Work out the finished part from the listing and answer in its coordinate system (mm). A direction names the side the tool comes from. Coordinates: 2 decimals unless noted, no trailing zeros. Loops run counter-clockwise (first coordinate to the right, second up) from the corner with the lowest first, then second, coordinate; pieces in that order, holes last. Notation, with made-up numbers: (35.25, 18.25) - (56.25, 18.25) arc R31 ccw to (56.25, 50.25) - close; hole circle Ø5 at (72, 0). An arc over 180 degrees is marked (long way). Write each question's results on one line, items separated by ' | '. Start each with the question number.
Item 1: Section A-A, the plane z = 37.5 is taken. Write down the section's boundary in (x, y).
Item 2: A tool of negligible diameter and unlimited length cuts with its end or side. For faces 4 (the face through (35, -13, 12.7)), 5 (the face through (6, -6.354, 38)), 6 (the face through (17, 0, 9)), from which of +Z, -Z, +X, -X, +Y, -Y can it reach the whole face along a straight path? Write none if from no direction.
Item 3: Consider probe 1 along X at (y, z) = (-11.75, 5); probe 2 along X at (y, z) = (-8, 8); probe 3 along Z at (x, y) = (34.5, -6.75). Determine where each line is inside the solid, lowest interval first. Write a range as [from, to].
Item 4: For a pull along Y with two mould halves and no side action, classify faces 1 (the face through (6, -19.046, 37)), 2 (the face through (6.439, -1.802, 38.489)), 3 (the face through (0, -13, 17)) as +Y half, -Y half, draft (parallel to the pull), parting line (faces both ways), or undercut.
Item 5: Section D-D, the plane x = 15.5 is taken. Write down the section's boundary in (y, z), plus the area to 3 significant figures.
Item 6: Section C-C, the plane z = 6 is taken. Write down the section's boundary in (x, y), plus the area to 3 significant figures.
Item 7: Each of these flat-tipped pins is pushed along its axis until it touches: pin 1 Ø4 at (y, z) = (-9, 18.5) entering from +X; pin 2 Ø12 at (x, z) = (6, 36.5) entering from -Y; pin 3 Ø5.5 at (x, z) = (5.5, 40) entering from +Y; pin 4 Ø8 at (y, z) = (-12.5, 37.5) entering from -X. Where does it stop, or does it pass through?
Item 8: Section B-B, the plane y = -11 is taken. Write down the section's boundary in (x, z), plus the area to 3 significant figures.
from build123d import *

# Parameters (mm, degrees)
F1_DEPTH = 25.4
F3_DEPTH = 12.701
F5_DEPTH = 12.701
F7_DEPTH = 57.151


with BuildPart() as f1:
    # F0 (on Front) → F1 (new body)
    with BuildSketch(Plane.XZ):
        Polygon((0, 44.45), (0, 0), (57.15, 0), (57.15, 12.7), (12.7, 12.7), (12.7, 44.45), align=None)
    extrude(amount=F1_DEPTH)

    # F2 (on face) → F3 (cut, through all)
    with BuildSketch(Plane.XY.offset(12.7)):
        with BuildLine():
            Line((25.4, -19.05), (25.4, -6.35))
            ThreePointArc((25.4, -6.35), (19.05, -12.7), (25.4, -19.05))
        make_face()
        with BuildLine():
            ThreePointArc((31.75, -12.7), (29.8901280605, -8.2098719395), (25.4, -6.35))
            Line((25.4, -6.35), (25.4, -19.05))
            ThreePointArc((25.4, -19.05), (29.8901280605, -17.1901280605), (31.75, -12.7))
        make_face()
        with BuildLine():
            Line((44.45, -19.05), (44.45, -6.35))
            ThreePointArc((44.45, -6.35), (38.1, -12.7), (44.45, -19.05))
        make_face()
        with BuildLine():
            ThreePointArc((50.8, -12.7), (48.9401280605, -8.2098719395), (44.45, -6.35))
            Line((44.45, -6.35), (44.45, -19.05))
            ThreePointArc((44.45, -19.05), (48.9401280605, -17.1901280605), (50.8, -12.7))
        make_face()
        with BuildLine():
            Line((57.15, 0), (44.45, 0))
            ThreePointArc((44.45, 0), (53.4302561211, -3.7197438789), (57.15, -12.7))
            Line((57.15, -12.7), (57.15, 0))
        make_face()
        with BuildLine():
            Line((57.15, -25.4), (57.15, -12.7))
            ThreePointArc((57.15, -12.7), (53.4302561211, -21.6802561211), (44.45, -25.4))
            Line((44.45, -25.4), (57.15, -25.4))
        make_face()
    extrude(amount=-F3_DEPTH, mode=Mode.SUBTRACT)

    # F4 (on face) → F5 (cut, through all)
    with BuildSketch(Plane.YZ.offset(12.7)):
        with BuildLine():
            ThreePointArc((-25.4, 32.1787146746), (-25.4018088896, 31.9643573373), (-25.4, 31.75))
            Line((-25.4, 31.75), (-25.4, 32.1787146746))
        make_face()
        with BuildLine():
            Line((0, 32.1787146746), (0, 31.75))
            ThreePointArc((0, 31.75), (0.0018088896, 31.9643573373), (0, 32.1787146746))
        make_face()
        with BuildLine():
            Line((-25.4, 44.45), (-25.4, 32.1787146746))
            ThreePointArc((-25.4, 32.1787146746), (-22.4029254465, 40.1612583888), (-15.0333830306, 44.45))
            Line((-15.0333830306, 44.45), (-25.4, 44.45))
        make_face()
        with BuildLine():
            ThreePointArc((-10.3666169694, 44.45), (-2.9970745535, 40.1612583888), (0, 32.1787146746))
            Line((0, 32.1787146746), (0, 44.45))
            Line((0, 44.45), (-10.3666169694, 44.45))
        make_face()
    extrude(amount=-F5_DEPTH, mode=Mode.SUBTRACT)

    # F6 (on face) → F7 (cut, through all)
    with BuildSketch(Plane(origin=(0, 0, 0), x_dir=(0, -1, 0), z_dir=(-1, 0, 0))):
        with BuildLine():
            Line((6.3536190682, 32.1787146746), (6.3536190682, 31.75))
            Line((6.3536190682, 31.75), (19.0463809318, 31.75))
            Line((19.0463809318, 31.75), (19.0463809318, 32.1787146746))
            ThreePointArc((19.0463809318, 32.1787146746), (12.7, 38.3143573373), (6.3536190682, 32.1787146746))
        make_face()
        with BuildLine():
            Line((19.0463809318, 31.75), (6.3536190682, 31.75))
            ThreePointArc((6.3536190682, 31.75), (12.7, 25.6143573373), (19.0463809318, 31.75))
        make_face()
        with BuildLine():
            ThreePointArc((6.3536190682, 32.1787146746), (6.35, 31.9643573373), (6.3536190682, 31.75))
            Line((6.3536190682, 31.75), (6.3536190682, 32.1787146746))
        make_face()
        with BuildLine():
            Line((19.0463809318, 32.1787146746), (19.0463809318, 31.75))
            ThreePointArc((19.0463809318, 31.75), (19.0490951685, 31.8571633942), (19.05, 31.9643573373))
            ThreePointArc((19.05, 31.9643573373), (19.0490951685, 32.0715512803), (19.0463809318, 32.1787146746))
        make_face()
        with BuildLine():
            Line((6.3536190682, 42.9670569213), (6.3536190682, 32.1787146746))
            ThreePointArc((6.3536190682, 32.1787146746), (12.7, 38.3143573373), (19.0463809318, 32.1787146746))
            Line((19.0463809318, 32.1787146746), (19.0463809318, 42.9670569213))
            ThreePointArc((19.0463809318, 42.9670569213), (17.1027668181, 43.8787013567), (15.0333830306, 44.45))
            Line((15.0333830306, 44.45), (10.3666169694, 44.45))
            ThreePointArc((10.3666169694, 44.45), (8.2972331819, 43.8787013567), (6.3536190682, 42.9670569213))
        make_face()
    extrude(amount=-F7_DEPTH, mode=Mode.SUBTRACT)


solid = f1.part
Answer key:
1) outline: (0, -24.13) - (12.7, -24.13) - (12.7, -19.05) - (0, -19.05) - close; (0, -6.35) - (12.7, -6.35) - (12.7, -1.27) - (0, -1.27) - close
2) face 4: +Z, +X, +Y, -Y | face 5: +Z, +X, -X | face 6: +Z, -Z, +X, -X, +Y
3) probe 1: x = [0, 19.12], [31.68, 38.17], [50.73, 57.11] | probe 2: x = [0, 21.13], [29.67, 40.18], [48.72, 56.25] | probe 3: z = [0, 12.7]
4) face 1: undercut | face 2: +Y half | face 3: draft
5) outline: (-25.4, 0) - (0, 0) - (0, 12.7) - (-25.4, 12.7) - close | area: 323 mm^2
6) outline: (0, -25.4) - (44.45, -25.4) arc R12.7 ccw to (44.45, 0) - (0, 0) - close; hole circle Ø12.7 at (25.4, -12.7); hole circle Ø12.7 at (44.45, -12.7) | area: 1,130 mm^2
7) pin 1: stops at x = 12.7 | pin 2: stops at y = -25.4 | pin 3: stops at y = -1.15 | pin 4: passes through
8) outline: (0, 0) - (19.28, 0) - (19.28, 12.7) - (12.7, 12.7) - (12.7, 25.85) - (0, 25.85) - close; (31.52, 0) - (38.33, 0) - (38.33, 12.7) - (31.52, 12.7) - close; (50.57, 0) - (57.04, 0) - (57.04, 12.7) - (50.57, 12.7) - close | area: 581 mm^2
